Build history of the part. All positions in model axes, mm. Face numbers are marked on the shaded views. A direction names the side the tool comes from. Coordinates: 2 decimals unless noted, no trailing zeros. Write each loop counter-clockwise with the first axis right and the second up, starting at its lowest first coordinate (ties: lowest second). Pieces come first, ordered by that corner, then holes.
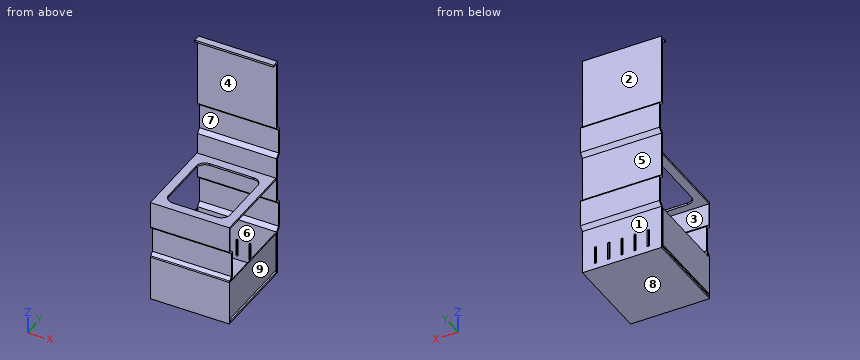
```python
from build123d import *

# Parameters (mm, degrees)
F0_W     = 96.8
F0_H     = 2.2
F0_W_2   = 2.2
F0_W_3   = 1
F0_W_4   = 5.8
F0_W_5   = 95.8395342231
F1_DEPTH = 90
F2_W     = 1
F2_H     = 45
F3_DEPTH = 96
F4_W     = 70
F4_H     = 76.8395342231
F5_DEPTH = 25
F6_R     = 10
F7_W     = 2.5
F7_H     = 20.3
F8_DEPTH = 25


# Not quite as in the source:
# - ends of sketch curves that miss each other by under 0.0002 mm in the source are joined


with BuildPart() as f1:
    # F0 (on Right) → F1 (new body)
    with BuildSketch(Plane.YZ):
        Polygon((-70.5190410137, 78.9974663137), (-66.1190410137, 74.5974663137), (-66.1190410137, 46.4200059881), (-70.5190410137, 42.0200059881), (-70.5190410137, -7.2912638491), (-68.3190410137, -7.2912638491), (-68.3190410137, 41.1087361509), (-63.9190410137, 45.5087361509), (-63.9190410137, 75.5087361509), (-68.3190410137, 79.9087361509), (-68.3190410137, 131.1087361509), (-63.9190410137, 135.5087361509), (-63.9190384975, 165.5087359606), (-68.3190385763, 169.9087361509), (-68.3190385763, 240.5087361509), (-68.3190385763, 248.3087361509), (-70.5190385763, 248.3087361509), (-70.5190385763, 238.3087361509), (-70.5190385763, 168.9974663137), (-66.1190385763, 164.5974663137), (-66.1190410137, 136.4200059881), (-70.5190410137, 132.0200059881), align=None)
        with Locations((-118.9190410137, -8.3912638491)):
            Rectangle(F0_W, F0_H)
        with Locations((-69.4190410137, -8.3912638491)):
            Rectangle(F0_W_2, F0_H)
        Polygon((-168.3190410137, -7.2912638491), (-167.3190410137, -7.2912638491), (-167.3190410137, 39.4887340454), (-168.3190410137, 38.4768152958), align=None)
        with Locations((-167.8190410137, -8.3912638491)):
            Rectangle(F0_W_3, F0_H)
        Polygon((-168.3190410137, 38.4768152958), (-167.3190410137, 39.4887340454), (-167.3190410137, 42.6143072478), (-168.3190410137, 41.6143048104), align=None)
        Polygon((-167.3190410137, 42.6143072478), (-167.3190410137, 39.4887340454), (-166.1190411219, 40.7030364356), (-161.7190464841, 45.1030417978), (-161.7190408009, 75.1030386029), (-166.1190410137, 79.5030349731), (-167.3190410137, 80.7030349731), (-167.3190410137, 77.5917651359), (-163.9190410137, 74.1917651359), (-163.9190475947, 46.0143089539), align=None)
        with Locations((-73.4190385763, 249.4087361509)):
            Rectangle(F0_W_4, F0_H)
        with Locations((-69.4190385763, 249.4087361509)):
            Rectangle(F0_W_2, F0_H)
        Polygon((-168.3190410137, 78.5917651359), (-167.3190410137, 77.5917651359), (-167.3190410137, 80.7030349731), (-168.3190410137, 81.7030349731), align=None)
        Polygon((-168.3190410137, 81.7030349731), (-167.3190410137, 80.7030349731), (-167.3190410137, 106.5323576331), (-168.3190410137, 106.5323576331), align=None)
        with Locations((-167.8190410137, 107.6323576331)):
            Rectangle(F0_W_3, F0_H)
        with Locations((-119.3992739022, 107.6323576331)):
            Rectangle(F0_W_5, F0_H)
    extrude(amount=F1_DEPTH)

    # F2 (on face) → F3 (join)
    with BuildSketch(Plane(origin=(0, -167.3190410137, 0), x_dir=(-1, 0, 0), z_dir=(0, 1, 0))):
        with Locations((-89.5, 18.2087361509)):
            Rectangle(F2_W, F2_H)
        with Locations((-0.5, 18.2087361509)):
            Rectangle(F2_W, F2_H)
    extrude(amount=F3_DEPTH)

    # F4 (on face) → F5 (cut)
    with BuildSketch(Plane.XY.offset(108.7323576331)):
        with Locations((45, -119.8992739022)):
            Rectangle(F4_W, F4_H)
    extrude(amount=-F5_DEPTH, mode=Mode.SUBTRACT)

    # F6
    f6_edges = [f1.edges().sort_by_distance(p)[0] for p in [
        (10, -81.479507, 107.632358),
        (10, -158.319041, 107.632358),
        (80, -81.479507, 107.632358),
        (80, -158.319041, 107.632358),
    ]]
    fillet(f6_edges, radius=F6_R)

    # F7 (on face) → F8 (cut)
    with BuildSketch(Plane(origin=(0, -68.3190410137, 0), x_dir=(-1, 0, 0), z_dir=(0, 1, 0))):
        with Locations((-75, 7.2530107699)):
            Rectangle(F7_W, F7_H)
        with Locations((-60, 7.2530107699)):
            Rectangle(F7_W, F7_H)
        with Locations((-45, 7.2530107699)):
            Rectangle(F7_W, F7_H)
        with Locations((-30, 7.2530107699)):
            Rectangle(F7_W, F7_H)
        with Locations((-15, 7.2530107699)):
            Rectangle(F7_W, F7_H)
    extrude(amount=-F8_DEPTH, mode=Mode.SUBTRACT)


solid = f1.part
```
1. Probe line 1 along Z through (x, y) = (84.5, -72.5); line 2 along Y through (x, z) = (67.5, 62.5); line 3 along Y through (x, z) = (55.5, 85.5). List the from-to ranges inside material, lowest first.
Computed values:
line 1: z = -9.49 to -7.29, 106.53 to 108.73, 248.31 to 250.51
line 2: y = -163.92 to -161.72, -66.12 to -63.92
line 3: y = -168.32 to -167.32, -70.52 to -68.32
2. Saw through at A-A on z = 29.5. List the corners of the cut face in (x, y).
Computed values:
outline: (0, -168.32) - (90, -168.32) - (90, -71.32) - (89, -71.32) - (89, -167.32) - (1, -167.32) - (1, -71.32) - (0, -71.32) - close; (0, -70.52) - (90, -70.52) - (90, -68.32) - (0, -68.32) - close
3. Flat gauge pins, fed straight in: pin 1 (10 mm diameter, centred on x = 29, z = 120.5, fed in from -Y); pin 2 (0.8 mm diameter, centred on x = 0.5, z = 7.5, fed in from +Y); pin 3 (0.7 mm diameter, centred on x = 33, z = 249, fed in from -Y). Where does each tip first touch, or does it go through?
Computed values:
pin 1: stops at y = -70.52
pin 2: stops at y = -68.32
pin 3: stops at y = -76.32
4. Saw through at C-C on z = 180.5. List the corners of the cut face in (x, y).
Computed values:
outline: (0, -70.52) - (90, -70.52) - (90, -68.32) - (0, -68.32) - close
5. Mould opens along Z. For the marked faces 6, 7, 8 and 9 say: +Z half, -Z half, draft (parallel to the pull), parting line (faces both ways), or undercut.
Computed values:
face 6: undercut
face 7: undercut
face 8: -Z half
face 9: draft
6. 3-axis set-ups, long thin cutter, end or side, ignore diameter. For the marked faces 1, 2, 3, 4 and 5: which of +Z, -Z, +X, -X, +Y, -Y reach the whole face in a straight line?
Computed values:
face 1: -Z, +X, -X, +Y
face 2: +Z, +X, -X, +Y
face 3: +X, -X
face 4: +X, -X, -Y
face 5: +X, -X, +Y
7. Saw through at B-B on y = -138.5. List the corners of the cut face in (x, z), plus the area to 3 significant figures.
Computed values:
outline: (0, -9.49) - (90, -9.49) - (90, -7.29) - (0, -7.29) - close; (0, -4.29) - (1, -4.29) - (1, 40.71) - (0, 40.71) - close; (0, 106.53) - (10, 106.53) - (10, 108.73) - (0, 108.73) - close; (80, 106.53) - (90, 106.53) - (90, 108.73) - (80, 108.73) - close; (89, -4.29) - (90, -4.29) - (90, 40.71) - (89, 40.71) - close
area: 332 mm2
